Build history of the part. All positions in model axes, mm. A direction names the side the tool comes from. Coordinates: 2 decimals unless noted, no trailing zeros. Write each loop counter-clockwise with the first axis right and the second up, starting at its lowest first coordinate (ties: lowest second). Pieces come first, ordered by that corner, then holes.
from build123d import *

# Parameters (mm, degrees)
F1_DEPTH      = 84
F2_W          = 31.5592023589
F2_H          = 27
F2_W_2        = 33.4407976411
F2_W_3        = 34
F2_H_2        = 25
F3_DEPTH      = 187.4
F5_DEPTH      = 299
F5_DEPTH_BACK = 323
F7_DEPTH      = 75.8


with BuildPart() as f1:
    # F0 (on Front) → F1 (new body)
    with BuildSketch(Plane.XZ):
        with BuildLine():
            Line((82, -43.5), (16.4407976411, 43.5))
            Line((16.4407976411, 43.5), (0, 43.5))
            Line((0, 43.5), (-82, 43.5))
            Line((-82, 43.5), (-82, -43.5))
            Line((-82, -43.5), (-70, -43.5))
            ThreePointArc((-70, -43.5), (-32, -5.5), (6, -43.5))
            Line((6, -43.5), (82, -43.5))
        make_face()
    extrude(amount=F1_DEPTH)

    # F2 (on face) → F3 (cut)
    with BuildSketch(Plane.XY.offset(43.5)):
        with Locations((32.2203988205, -40.5)):
            Rectangle(F2_W, F2_H)
        with Locations((-0.2796011795, -40.5)):
            Rectangle(F2_W_2, F2_H)
        with Locations((-65, -26.5)):
            Rectangle(F2_W_3, F2_H_2)
    extrude(amount=-F3_DEPTH, mode=Mode.SUBTRACT)

    # F4 (on Right) → F5 (cut, two sides)
    with BuildSketch(Plane.YZ) as f5_sk:
        Polygon((-84, -43.5), (-60.6884202585, 43.5), (-84, 43.5), align=None)
    extrude(amount=F5_DEPTH, mode=Mode.SUBTRACT)
    extrude(f5_sk.sketch, amount=-F5_DEPTH_BACK, mode=Mode.SUBTRACT)

    # F6 (on Top) → F7 (cut)
    with BuildSketch(Plane.XY):
        Polygon((82, -84), (48.8038917131, -72.1961082869), (37, -84), align=None)
        Polygon((82, -39), (48.8038917131, -72.1961082869), (82, -84), align=None)
    extrude(amount=-F7_DEPTH, mode=Mode.SUBTRACT)


solid = f1.part
(1) Probe L1, parallel to X at y = -29, z = 18; L2, parallel to X at y = -42, z = 28; L3, parallel to X at y = -30.5, z = -3.5. List the from-to ranges inside material, lowest first.
(2) Slice it at D-D, the plane z = -16. List the corners of the cut face in (x, y), and give its area (3 significant figures).
(3) Slice it at B-B, the plane z = -34. List the corners of the cut face in (x, y), and give its area (3 significant figures).
(4) Slice it at A-A, the plane x = 28.5. List the corners of the cut face in (y, z).
(5) Flat gauge pins, fed straight in: P1, Ø6, axis at y = -72.5, z = 10, coming from the +X side; P2, Ø2, axis at x = -12, y = -75, coming from the -Z side; P3, Ø10, axis at x = -58, z = 7.5, coming from the -Y side. Where does each tip first touch, or does it go through?
(6) Two-plate mould, pull along Y, no slides. Class faces 4 (the flat face through (55, -66, -31)), 5 (the flat face through (16, -27, 1)), 6 (the flat face through (52, -32, -43.5)): pulls with the +Y half, pulls with the -Y half, needs draft (parallel to the pull), parting line crosses it, or undercut.
(7) Slice it at C-C, the plane x = -54. List the corners of the cut face in (y, z).
(8) 3-axis set-ups, long thin cutter, end or side, ignore diameter. For faces 1 (the cylindrical face through (-32.84, -41.41, -5.51)), 2 (the flat face through (-17, -41, 18)), 3 (the flat face through (-65, -39, 10)): which of +Z, -Z, +X, -X, +Y, -Y reach the whole face in a straight line?
Results:
1. L1: x = -48 to -17
1. L2: x = -82 to -17
1. L3: x = -48 to -17, 48 to 51.86
2. outline: (-82, -76.63) - (-58.22, -76.63) - (-58.22, -39) - (-82, -39) - close; (-82, -14) - (-58.22, -14) - (-58.22, 0) - (-82, 0) - close; (-5.78, -76.63) - (44.37, -76.63) - (61.28, -59.72) - (61.28, 0) - (-5.78, 0) - (-5.78, -27) - (48, -27) - (48, -54) - (-5.78, -54) - close
2. area: 4,770 mm2
3. outline: (-82, -81.45) - (-68.79, -81.45) - (-68.79, -39) - (-82, -39) - close; (-82, -14) - (-68.79, -14) - (-68.79, 0) - (-82, 0) - close; (4.79, -81.45) - (39.55, -81.45) - (74.84, -46.16) - (74.84, 0) - (4.79, 0) - (4.79, -27) - (48, -27) - (48, -54) - (4.79, -54) - close
3. area: 4,660 mm2
4. outline: (-84, -43.5) - (-54, -43.5) - (-54, 27.5) - (-64.98, 27.5) - close; (-27, -43.5) - (0, -43.5) - (0, 27.5) - (-27, 27.5) - close
5. P1: stops at x = 43.11
5. P2: stops at z = -11.83
5. P3: stops at y = -71.67
6. face 4: pulls with the -Y half
6. face 5: undercut
6. face 6: needs draft
7. outline: (-75.7, -12.52) - (-39, -12.52) - (-39, 43.5) - (-60.69, 43.5) - close; (-14, -12.52) - (0, -12.52) - (0, 43.5) - (-14, 43.5) - close
8. face 1: -Z, +Y, -Y
8. face 2: +Z, -Z
8. face 3: +Z, -Z, -X
